```python
from build123d import *

# Parameters (mm, degrees)
SKETCH1_W           = 60
SKETCH1_H           = 50
BOSS_EXTRUDE1_DEPTH = 12
SKETCH2_R           = 11
CUT_EXTRUDE1_DEPTH  = 4
CUT_EXTRUDE5_REACH  = 41.862
SKETCH6_R           = 12
CUT_EXTRUDE7_DEPTH  = 8
CUT_EXTRUDE8_DEPTH  = 6.5
FILLET1_R           = 10


with BuildPart() as part:
    # Sketch1 → Boss-Extrude1 (new body)
    with BuildSketch(Plane.XY):
        Rectangle(SKETCH1_W, SKETCH1_H)
    extrude(amount=BOSS_EXTRUDE1_DEPTH)

    # Sketch2 → Cut-Extrude1 (cut)
    with BuildSketch(Plane.XY.offset(12)):
        with Locations((0, 4.5)):
            Circle(SKETCH2_R)
    extrude(amount=-CUT_EXTRUDE1_DEPTH, mode=Mode.SUBTRACT)

    # Sketch6 → Cut-Extrude5 (cut, up to next)
    with BuildSketch(Plane.XY.offset(8), mode=Mode.PRIVATE) as cut_extrude5_sk1:
        with Locations((0, 4.5)):
            Circle(SKETCH6_R)
    cut_extrude5_tool1 = extrude(cut_extrude5_sk1.sketch, amount=-CUT_EXTRUDE5_REACH, mode=Mode.PRIVATE) & part.part
    add(cut_extrude5_tool1.solids().sort_by_distance((0, 4.5, 8))[0], mode=Mode.SUBTRACT)

    # Sketch9 → Cut-Extrude7 (cut)
    with BuildSketch(Plane(origin=(33.355171667, 100.110949441, 0), x_dir=(-1, 0, 0), z_dir=(0, 0, -1))):
        with BuildLine():
            Line((9.355171667, -111.110949441), (17.355171667, -111.110949441))
            ThreePointArc((17.355171667, -111.110949441), (19.355171667, -113.110949441), (17.355171667, -115.110949441))
            Line((17.355171667, -115.110949441), (9.355171667, -115.110949441))
            ThreePointArc((9.355171667, -115.110949441), (7.355171667, -113.110949441), (9.355171667, -111.110949441))
        make_face()
    cut_extrude7 = extrude(amount=-CUT_EXTRUDE7_DEPTH, mode=Mode.SUBTRACT)

    # Sketch11 → Cut-Extrude8 (cut)
    with BuildSketch(Plane(origin=(33.355171667, 100.110949441, 0), x_dir=(-1, 0, 0), z_dir=(0, 0, -1))):
        with BuildLine():
            Line((15.855171667, -108.110949441), (15.855171667, -132.025405836))
            ThreePointArc((15.855171667, -132.025405836), (13.355171667, -134.525405836), (10.855171667, -132.025405836))
            Line((10.855171667, -132.025405836), (10.855171667, -108.110949441))
            ThreePointArc((10.855171667, -108.110949441), (13.355171667, -105.610949441), (15.855171667, -108.110949441))
        make_face()
    cut_extrude8 = extrude(amount=-CUT_EXTRUDE8_DEPTH, mode=Mode.SUBTRACT)

    # Mirror1: Cut-Extrude7, Cut-Extrude8 across plane
    add(cut_extrude7.mirror(Plane(origin=(0, 0, 0), x_dir=(0, 0, 1), z_dir=(1, 0, 0))), mode=Mode.SUBTRACT)
    add(cut_extrude8.mirror(Plane(origin=(0, 0, 0), x_dir=(0, 0, 1), z_dir=(1, 0, 0))), mode=Mode.SUBTRACT)

    # Fillet1
    fillet1_edges = [part.edges().sort_by_distance(p)[0] for p in [
        (-30, 25, 6),
        (30, 25, 6),
    ]]
    fillet(fillet1_edges, radius=FILLET1_R)


solid = part.part
```
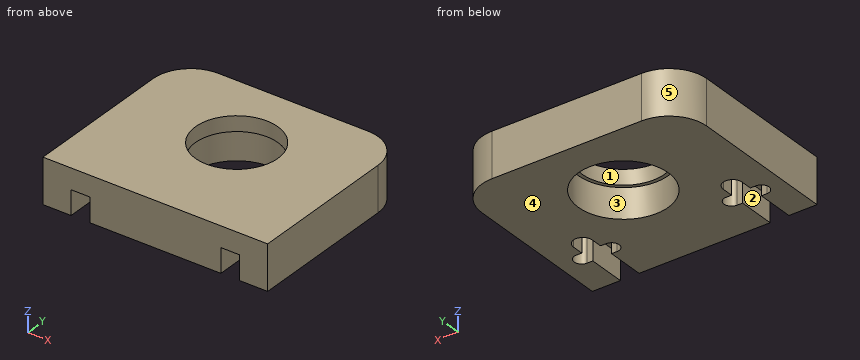
Check sheet for the modelled part. Datum: model origin and axes. Units: mm. Face numbers are marked on the shaded views. A direction names the side the tool comes from. Coordinates: 2 decimals unless noted, no trailing zeros. Order: outer loops, then holes, each group sorted by start corner. A loop starts at its lowest first (then second) coordinate and runs counter-clockwise, first axis right, second up. Notation, with made-up numbers: (39.25, 77.5) -> (56.25, 77.5) arc R26 ccw to (56.25, 107.5) -> close; hole circle Ø6 at (-14.75, 77.25). An arc over 180 degrees is marked (long way). Write item = value, one per line. Start each with the question number.
1) Go/stop test with flat-tipped pins: P1, Ø1.5, axis at x = 21, y = -7.5, coming from the -Z side; P2, Ø12, axis at x = 5.5, y = 5, coming from the -Z side; P3, Ø1, axis at y = 17.5, z = 2, coming from the -X side. Record where each tip stops, or that it passes through.
2) Cross-section at C-C (y = 1.5). Enter the section's corners in (x, z).
3) Cross-section at D-D (y = -19.5). Enter the section's corners in (x, z), then the cut area to 3 significant figures.
4) Mould release check, pull along Y, two halves, no side actions. Record for the marked faces 3, 4 and 5: +Y half, -Y half, draft (parallel to the pull), parting line (faces both ways), or undercut.
5) Cross-section at B-B (x = 0). Enter the section's corners in (y, z), then the cut area to 3 significant figures.
6) Material ranges on L1, parallel to X at y = -18, z = 4.25; L2, parallel to Y at x = 0, z = 6.25; L3, parallel to X at y = -11.5, z = 6.5, recorded low to high.
7) Access from +Z, -Z, +X, -X, +Y, -Y to the whole of each face (thin tool, end or side, straight path). Record for the marked faces 1 and 2.
8) Cross-section at A-A (z = 9.5). Enter the section's corners in (x, y).
Ans:
q1.P1 = 6.5
q1.P2 = 8
q1.P3 = -29.8
q2.outline = (-30, 0) -> (-11.62, 0) -> (-11.62, 8) -> (-10.58, 8) -> (-10.58, 12) -> (-30, 12) -> close; (10.58, 8) -> (11.62, 8) -> (11.62, 0) -> (30, 0) -> (30, 12) -> (10.58, 12) -> close
q3.outline = (-30, 0) -> (-22.5, 0) -> (-22.5, 6.5) -> (-17.5, 6.5) -> (-17.5, 0) -> (17.5, 0) -> (17.5, 6.5) -> (22.5, 6.5) -> (22.5, 0) -> (30, 0) -> (30, 12) -> (-30, 12) -> close
q3.area = 655 mm²
q4.face_3 = undercut
q4.face_4 = draft
q4.face_5 = +Y half
q5.outline = (-25, 0) -> (-7.5, 0) -> (-7.5, 8) -> (-6.5, 8) -> (-6.5, 12) -> (-25, 12) -> close; (15.5, 8) -> (16.5, 8) -> (16.5, 0) -> (25, 0) -> (25, 12) -> (15.5, 12) -> close
q5.area = 320 mm²
q6.L1 = -30 to -22.5, -17.5 to 17.5, 22.5 to 30
q6.L2 = -25 to -7.5, 16.5 to 25
q6.L3 = -30 to -25.32, -14.68 to 14.68, 25.32 to 30
q7.face_1 = +Z, -Z
q7.face_2 = -Z, -Y
q8.outline = (-30, -25) -> (30, -25) -> (30, 15) arc R10 ccw to (20, 25) -> (-20, 25) arc R10 ccw to (-30, 15) -> close; hole circle Ø22 at (0, 4.5)
